from build123d import *

# Parameters (mm, degrees)
SKETCH1_R                       = 100
BOSS_EXTRUDE1_DEPTH             = 15
BOSS_EXTRUDE2_DEPTH             = 75
BOSS_EXTRUDE2_DIRECTION_2_REACH = 144.215
SKETCH3_W                       = 85
SKETCH3_H                       = 120
CUT_EXTRUDE1_DEPTH              = 62.8
SKETCH4_W                       = 20
SKETCH4_H                       = 55
CUT_EXTRUDE2_DEPTH              = 5
SKETCH5_R                       = 30
BOSS_EXTRUDE3_DEPTH             = 2.5
SKETCH6_R                       = 17.5
BOSS_EXTRUDE4_DEPTH             = 15
BOSS_EXTRUDE5_DEPTH             = 5
BOSS_EXTRUDE5_DIRECTION_2_REACH = 163.942
SKETCH8_R                       = 6
CUT_EXTRUDE3_DEPTH              = 20
SKETCH11_R                      = 5
CUT_EXTRUDE4_DEPTH              = 15


with BuildPart() as part:
    # Sketch1 → Boss-Extrude1 (new body)
    with BuildSketch(Plane(origin=(0, 0, 0), x_dir=(1, 0, 0), z_dir=(0, 1, 0))):
        with Locations(Location((0, 0, 0), (0, 0, 270))):
            Circle(SKETCH1_R)
    extrude(amount=BOSS_EXTRUDE1_DEPTH)

    # Sketch2 → Boss-Extrude2 (add)
    with BuildSketch(Plane(origin=(0, 15, 0), x_dir=(1, 0, 0), z_dir=(0, 1, 0))):
        Polygon((-2.5, 52.043156662), (-2.5, 39.543156662), (-72.5, 39.543156662), (-72.5, -90.456843338), (-2.5, -90.456843338), (-2.5, -102.956843338), (17.5, -102.956843338), (17.5, 52.043156662), align=None)
    extrude(amount=BOSS_EXTRUDE2_DEPTH)

    # Boss-Extrude2 direction 2: up to this face of the body (flat: up to its plane)
    boss_extrude2_direction_2_end = Plane(part.part.faces().sort_by_distance((0, 0, 0))[0])
    # Sketch2 → Boss-Extrude2 direction 2 (add, up to the picked face)
    with BuildSketch(Plane(origin=(0, 15, 0), x_dir=(1, 0, 0), z_dir=(0, 1, 0)), mode=Mode.PRIVATE) as boss_extrude2_direction_2_sk1:
        Polygon((-2.5, 52.043156662), (-2.5, 39.543156662), (-72.5, 39.543156662), (-72.5, -90.456843338), (-2.5, -90.456843338), (-2.5, -102.956843338), (17.5, -102.956843338), (17.5, 52.043156662), align=None)
    boss_extrude2_direction_2_tool1 = split(extrude(boss_extrude2_direction_2_sk1.sketch, amount=-BOSS_EXTRUDE2_DIRECTION_2_REACH, mode=Mode.PRIVATE), bisect_by=boss_extrude2_direction_2_end, keep=Keep.BOTH, mode=Mode.PRIVATE)
    add(boss_extrude2_direction_2_tool1.solids().sort_by(Axis((-26.065574, 15, 25.456843), (0, -1, 0)))[0])

    # Sketch3 → Cut-Extrude1 (cut)
    with BuildSketch(Plane(origin=(0, 90, 0), x_dir=(1, 0, 0), z_dir=(0, 1, 0))):
        with Locations((-25, -25.456843338)):
            Rectangle(SKETCH3_W, SKETCH3_H)
    extrude(amount=-CUT_EXTRUDE1_DEPTH, mode=Mode.SUBTRACT)

    # Sketch4 → Cut-Extrude2 (cut)
    with BuildSketch(Plane.XY.offset(90.456843338)):
        with Locations((-31.7, 62.5)):
            Rectangle(SKETCH4_W, SKETCH4_H)
    extrude(amount=-CUT_EXTRUDE2_DEPTH, mode=Mode.SUBTRACT)

    # Sketch5 → Boss-Extrude3 (add)
    with BuildSketch(Plane.ZY.offset(72.5)):
        with Locations(Location((52.956843338, 60, 0), (0, 0, 90))):
            Circle(SKETCH5_R)
    extrude(amount=BOSS_EXTRUDE3_DEPTH)

    # Sketch6 → Boss-Extrude4 (add)
    with BuildSketch(Plane.ZY.offset(75)):
        with Locations((52.956843338, 60)):
            Circle(SKETCH6_R)
    extrude(amount=BOSS_EXTRUDE4_DEPTH)

    # Sketch7 → Boss-Extrude5 (add)
    with BuildSketch(Plane(origin=(0, 15, 0), x_dir=(1, 0, 0), z_dir=(0, 1, 0))):
        with BuildLine():
            Line((63.042469592, 37.893156662), (92.542469592, 37.893156662))
            ThreePointArc((92.542469592, 37.893156662), (85.873522386, 51.24195696), (77.292469592, 63.449776551))
            Line((77.292469592, 63.449776551), (77.292469592, 113.371099331))
            Line((77.292469592, 113.371099331), (67.292469592, 113.371099331))
            Line((67.292469592, 113.371099331), (67.292469592, 73.971099331))
            ThreePointArc((67.292469592, 73.971099331), (65.19307414, 75.827851639), (63.042469592, 77.625041242))
            Line((63.042469592, 77.625041242), (63.042469592, 37.893156662))
        make_face()
    extrude(amount=BOSS_EXTRUDE5_DEPTH)

    # Boss-Extrude5 direction 2: up to this face of the body (flat: up to its plane)
    boss_extrude5_direction_2_end = Plane(part.part.faces().sort_by_distance((-0.54005377, 0, 0.955561691))[0])
    # Sketch7 → Boss-Extrude5 direction 2 (add, up to the picked face)
    with BuildSketch(Plane(origin=(0, 15, 0), x_dir=(1, 0, 0), z_dir=(0, 1, 0)), mode=Mode.PRIVATE) as boss_extrude5_direction_2_sk1:
        with BuildLine():
            Line((63.042469592, 37.893156662), (92.542469592, 37.893156662))
            ThreePointArc((92.542469592, 37.893156662), (85.873522386, 51.24195696), (77.292469592, 63.449776551))
            Line((77.292469592, 63.449776551), (77.292469592, 113.371099331))
            Line((77.292469592, 113.371099331), (67.292469592, 113.371099331))
            Line((67.292469592, 113.371099331), (67.292469592, 73.971099331))
            ThreePointArc((67.292469592, 73.971099331), (65.19307414, 75.827851639), (63.042469592, 77.625041242))
            Line((63.042469592, 77.625041242), (63.042469592, 37.893156662))
        make_face()
    boss_extrude5_direction_2_tool1 = split(extrude(boss_extrude5_direction_2_sk1.sketch, amount=-BOSS_EXTRUDE5_DIRECTION_2_REACH, mode=Mode.PRIVATE), bisect_by=boss_extrude5_direction_2_end, keep=Keep.BOTH, mode=Mode.PRIVATE)
    add(boss_extrude5_direction_2_tool1.solids().sort_by(Axis((73.261773, 15, -67.454705), (0, -1, 0)))[0])

    # Sketch8 → Cut-Extrude3 (cut)
    with BuildSketch(Plane(origin=(17.5, 0, 0), x_dir=(0, 0, -1), z_dir=(1, 0, 0))):
        with Locations((-92.931843338, 55)):
            Circle(SKETCH8_R)
        with Locations(Location((42.018156662, 55, 0), (0, 0, 245.63802206))):
            Circle(SKETCH8_R)
    extrude(amount=-CUT_EXTRUDE3_DEPTH, mode=Mode.SUBTRACT)

    # Sketch11 → Cut-Extrude4 (cut)
    with BuildSketch(Plane.XZ):
        with Locations(Location((-30.0520382, 30.0520382, 0), (0, 0, 270))):
            Circle(SKETCH11_R)
        with Locations(Location((30.0520382, 30.0520382, 0), (0, 0, 270))):
            Circle(SKETCH11_R)
        with Locations(Location((30.0520382, -30.0520382, 0), (0, 0, 270))):
            Circle(SKETCH11_R)
        with Locations(Location((-30.0520382, -30.0520382, 0), (0, 0, 270))):
            Circle(SKETCH11_R)
    extrude(amount=-CUT_EXTRUDE4_DEPTH, mode=Mode.SUBTRACT)


solid = part.part
Can you work these out from the model? Positions are in its coordinate system, mm. A direction names the side the tool comes from. Give positions to 0.01 mm unless a question says otherwise; leave off trailing zeros. Loops run counter-clockwise (first coordinate to the right, second up) from the corner with the lowest first, then second, coordinate; pieces in that order, holes last. Notation, with made-up numbers: (18, 40.25) - (72, 40.25) arc R29 cw to (72, 77.25) - close; hole circle Ø4 at (87.5, 78). An arc over 180 degrees is marked (long way). One line per item, written item: value.
(1) I need wall thicknesses on line 1 along Z through (x, y) = (9.75, 55); line 2 along Z through (x, y) = (-13.5, 61); line 3 along X through (y, z) = (54, 86.5). Which ranges of each line are inside material? Lowest first, please.
Verdict:
line 1: -52.04 to -48.02, -36.02 to -34.54, 85.46 to 86.93, 98.93 to 102.96
line 2: -39.54 to -34.54, 85.46 to 90.46
line 3: -72.5 to -41.7, -21.7 to 17.5
(2) If we section it at C-C, the plane y = 55: State how many separate pieces and enclosed holes the cut face has, plus the area to 3 significant figures.
Verdict:
separate pieces: 4
enclosed holes: 0
area: 2,070 mm^2
(3) I'm going to push flat-ended pins straight in: pin 1 (8 mm diameter, centred on x = 5, z = 80, fed in from -Y); pin 2 (2 mm diameter, centred on y = 9.5, z = -84, fed in from -X); pin 3 (22 mm diameter, centred on y = 10, z = -99.5, fed in from -X); pin 4 (2 mm diameter, centred on y = 12.5, z = -84.5, fed in from +X). Where does each tip first touch, or does it pass through?
Verdict:
pin 1: y = 0
pin 2: x = -55.78
pin 3: x = -46.56
pin 4: x = 77.29
(4) If we section it at D-D, the plane y = 72.5: List the corners of the cut face in (x, z) for me, plus the area to 3 significant figures.
Verdict:
outline: (-90, 40.71) - (-75, 40.71) - (-75, 25.69) - (-72.5, 25.69) - (-72.5, -39.54) - (-2.5, -39.54) - (-2.5, -52.04) - (17.5, -52.04) - (17.5, -34.54) - (-67.5, -34.54) - (-67.5, 85.46) - (-41.7, 85.46) - (-41.7, 90.46) - (-72.5, 90.46) - (-72.5, 80.23) - (-75, 80.23) - (-75, 65.2) - (-90, 65.2) - close; (-21.7, 85.46) - (17.5, 85.46) - (17.5, 102.96) - (-2.5, 102.96) - (-2.5, 90.46) - (-21.7, 90.46) - close
area: 2,400 mm^2
(5) If we section it at A-A, the plane x = 0: List the corners of the cut face in (y, z) for me, plus the area to 3 significant figures.
Verdict:
outline: (0, -100) - (15, -100) - (15, -52.04) - (90, -52.04) - (90, -34.54) - (27.2, -34.54) - (27.2, 85.46) - (90, 85.46) - (90, 102.96) - (0, 102.96) - close; hole circle Ø12 at (55, -42.02); hole circle Ø12 at (55, 92.93)
area: 6,910 mm^2
(6) If we mould it in two halves opening along Z, with no side actions, what happens to faces 1 (the face through (34.27, 7.4, -32.74)), 2 (the face through (-37, 52, -39.543)), 3 (the face through (63.042, 17, -58))? For each: released by +Z, released by -Z, zero draft, split by the parting line, or undercut.
Verdict:
face 1: undercut
face 2: released by -Z
face 3: zero draft
(7) If we section it at B-B, the plane z = -28.5: List the corners of the cut face in (x, y) for me, plus the area to 3 significant figures.
Verdict:
outline: (-95.85, 0) - (-34.81, 0) - (-34.81, 15) - (-25.3, 15) - (-25.3, 0) - (25.3, 0) - (25.3, 15) - (17.5, 15) - (17.5, 27.2) - (-67.5, 27.2) - (-67.5, 90) - (-72.5, 90) - (-72.5, 15) - (-95.85, 15) - close; (34.81, 0) - (95.85, 0) - (95.85, 15) - (34.81, 15) - close
area: 4,000 mm^2
(8) On a 3-axis mill with a long thin cutter (end or side, diameter ignored), from which of +Z, -Z, +X, -X, +Y, -Y can I reach the whole of each face in a straight line? I mean faces 4 (the face through (78, 17, -37.893)), 5 (the face through (-41.7, 62, 88)), 6 (the face through (7.64, 55.264, 98.926)). Say none if no direction works.
Verdict:
face 4: +Z, +X, +Y
face 5: +Z, +Y
face 6: +X
